from build123d import *

# Parameters (mm, degrees)
SKETCH1_R           = 31
SKETCH1_R_2         = 25
BOSS_EXTRUDE1_DEPTH = 6
SKETCH2_R           = 29
SKETCH2_R_2         = 27
CUT_EXTRUDE1_DEPTH  = 1
SKETCH3_R           = 29
SKETCH3_R_2         = 27
CUT_EXTRUDE2_DEPTH  = 1


with BuildPart() as part:
    # Sketch1 → Boss-Extrude1 (new body)
    with BuildSketch(Plane(origin=(0, 0, 0), x_dir=(1, 0, 0), z_dir=(0, 1, 0))):
        Circle(SKETCH1_R)
        Circle(SKETCH1_R_2, mode=Mode.SUBTRACT)
    extrude(amount=BOSS_EXTRUDE1_DEPTH)

    # Sketch2 → Cut-Extrude1 (cut)
    with BuildSketch(Plane(origin=(0, 6, 0), x_dir=(1, 0, 0), z_dir=(0, 1, 0))):
        Circle(SKETCH2_R)
        Circle(SKETCH2_R_2, mode=Mode.SUBTRACT)
    extrude(amount=-CUT_EXTRUDE1_DEPTH, mode=Mode.SUBTRACT)

    # Sketch3 → Cut-Extrude2 (cut)
    with BuildSketch(Plane.XZ):
        Circle(SKETCH3_R)
        Circle(SKETCH3_R_2, mode=Mode.SUBTRACT)
    extrude(amount=-CUT_EXTRUDE2_DEPTH, mode=Mode.SUBTRACT)


solid = part.part
Verification items for the finished model (mm, model axes). A direction names the side the tool comes from. Give positions to 0.01 mm unless a question says otherwise; leave off trailing zeros. Loops run counter-clockwise (first coordinate to the right, second up) from the corner with the lowest first, then second, coordinate; pieces in that order, holes last.
1) Depth check by flat-ended pin: pin 1 Ø1 at (y, z) = (4.5, -1) entering from +X. Enter the tip coordinate at first touch or a pass-through.
2) Sectioned sample at B-B, the plane z = 0. Enter the section's corners in (x, y), then the cut area to 3 significant figures.
3) Set-up check for faces 4 (the cylindrical face through (13.38, 0.49, -25.73)), 5 (the cylindrical face through (13.38, 5.51, 25.73)), 6 (the flat face through (21, 0, 21)): record each of +Z, -Z, +X, -X, +Y, -Y from which the full face is reachable in a straight line by a thin tool's end or side.
4) Thickness scan on line 1 along Z through (x, y) = (0, 5.35); line 2 along Z through (x, y) = (0, 3.9); line 3 along X through (y, z) = (0.7, 21). Record the ranges inside material, lowest first.
5) Sectioned sample at D-D, the plane x = 26. Enter the section's corners in (y, z).
6) Sectioned sample at A-A, the plane x = 0. Enter the section's corners in (y, z).
7) Sectioned sample at C-C, the plane y = 2. Enter the section's corners in (x, z).
8) Draft check along X on faces 1 (the cylindrical face through (-4.036, 2.958, -30.736)), 2 (the flat face through (24, 0, 8)), 3 (the flat face through (8, 1, -26)). Enter one of: pulls with the +X half, pulls with the -X half, needs draft (parallel to the pull), parting line crosses it, or undercut.
Answers:
1. pin 1: stops at x = 31
2. outline: (-31, 0) - (-29, 0) - (-29, 1) - (-27, 1) - (-27, 0) - (-25, 0) - (-25, 6) - (-27, 6) - (-27, 5) - (-29, 5) - (-29, 6) - (-31, 6) - close; (25, 0) - (27, 0) - (27, 1) - (29, 1) - (29, 0) - (31, 0) - (31, 6) - (29, 6) - (29, 5) - (27, 5) - (27, 6) - (25, 6) - close
2. area: 64.0 mm2
3. face 4: -Y
3. face 5: +Y
3. face 6: +Z, -Z, +X, -X, -Y
4. line 1: z = -31 to -29, -27 to -25, 25 to 27, 29 to 31
4. line 2: z = -31 to -25, 25 to 31
4. line 3: x = -22.8 to -20, -16.97 to -13.56, 13.56 to 16.97, 20 to 22.8
5. outline: (0, -16.88) - (6, -16.88) - (6, -12.85) - (5, -12.85) - (5, -7.28) - (6, -7.28) - (6, 7.28) - (5, 7.28) - (5, 12.85) - (6, 12.85) - (6, 16.88) - (0, 16.88) - (0, 12.85) - (1, 12.85) - (1, 7.28) - (0, 7.28) - (0, -7.28) - (1, -7.28) - (1, -12.85) - (0, -12.85) - close
6. outline: (0, -31) - (6, -31) - (6, -29) - (5, -29) - (5, -27) - (6, -27) - (6, -25) - (0, -25) - (0, -27) - (1, -27) - (1, -29) - (0, -29) - close; (0, 25) - (6, 25) - (6, 27) - (5, 27) - (5, 29) - (6, 29) - (6, 31) - (0, 31) - (0, 29) - (1, 29) - (1, 27) - (0, 27) - close
7. outline: circle Ø62 at (0, 0); hole circle Ø50 at (0, 0)
8. face 1: parting line crosses it
8. face 2: needs draft
8. face 3: undercut
